Work out the finished part from the listing and answer in its coordinate system (mm). Face numbers are marked on the shaded views. A direction names the side the tool comes from. Coordinates: 2 decimals unless noted, no trailing zeros. Loops run counter-clockwise (first coordinate to the right, second up) from the corner with the lowest first, then second, coordinate; pieces in that order, holes last. Notation, with made-up numbers: M 64,63 L 114,63 A34 cw 114,98 Z; hole C -33.75,10.5 d3. An arc over 180 degrees is marked long. Write each question's results on one line, items separated by ' | '.
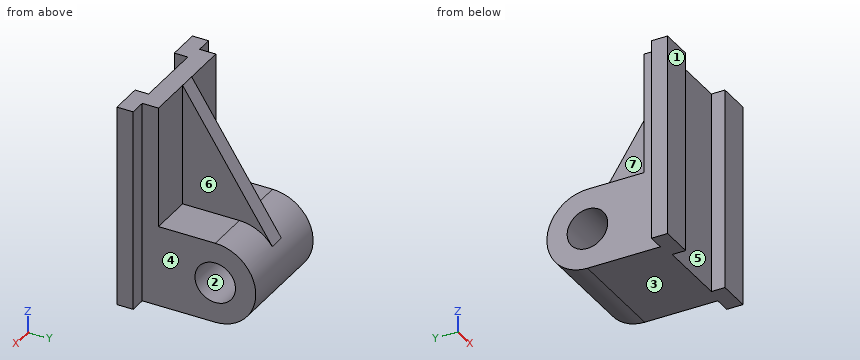
```python
from build123d import *

# Parameters (mm, degrees)
BOSS_EXTRUDE1_DEPTH = 150
SKETCH4_R           = 15
BOSS_EXTRUDE2_DEPTH = 38
RIB1_REACH          = 181.042
SKETCH5_WALL_W      = 482.19756146
SKETCH5_WALL_H      = 12


with BuildPart() as part:
    # Sketch1 → Boss-Extrude1 (new body)
    with BuildSketch(Plane.XY):
        Polygon((-50, 0), (-38, 0), (-38, 12), (38, 12), (38, 0), (50, 0), (50, -12), (26, -12), (26, -2), (-26, -2), (-26, -12), (-50, -12), align=None)
    extrude(amount=BOSS_EXTRUDE1_DEPTH)

    # Sketch4 → Boss-Extrude2 (add, symmetric)
    with BuildSketch(Plane(origin=(0, 0, 0), x_dir=(0, 0, -1), z_dir=(1, 0, 0))):
        with BuildLine():
            Line((0, 12), (0, 54))
            ThreePointArc((0, 54), (-30, 84), (-60, 54))
            Line((-60, 54), (-60, 12))
            Line((-60, 12), (0, 12))
        make_face()
        with Locations((-30, 54)):
            Circle(SKETCH4_R, mode=Mode.SUBTRACT)
    extrude(amount=BOSS_EXTRUDE2_DEPTH, both=True)

    # Sketch5 wall → Rib1 (add, up to next)
    with BuildSketch(Plane(origin=(0, 45.18462462, 98.748424022), x_dir=(0, 0.54350338987, -0.839406972332), z_dir=(0, 0.839406972332, 0.54350338987)), mode=Mode.PRIVATE) as rib1_sk1:
        Rectangle(SKETCH5_WALL_W, SKETCH5_WALL_H)
    rib1_tool1 = extrude(rib1_sk1.sketch, amount=-RIB1_REACH, mode=Mode.PRIVATE) - part.part
    add(rib1_tool1.solids().sort_by_distance((0, 45.18462462, 98.748424022))[0])


solid = part.part
```
1) Find section A-A, the plane x = -35. Give the vertices of the cut face in (y, z).
Check result:
outline: M -12,0 L 54,0 A30 ccw 54,60 L 12,60 L 12,150 L -12,150 Z; hole C 54,30 d30
2) Find section D-D, the plane x = 3. Give the vertices of the cut face in (y, z).
Check result:
outline: M -2,0 L 54,0 A30 ccw 78.37,47.5 L 12,150 L -2,150 Z; hole C 54,30 d30
3) Given pin 1 Ø18 at (y, z) = (54, 30) entering from -X; pin 2 Ø2 at (y, z) = (38.5, 95) entering from +X; pin 3 Ø3 at (x, y) = (-25, 32) entering from +Z; pin 4 Ø4 at (x, z) = (-15, 86.5) entering from -Y, each flat-ended and moving along its own axis, determine where each tip first touches the part or whether it passes through.
Check result:
pin 1: through | pin 2: x = 6 | pin 3: z = 60 | pin 4: y = -2
4) For a pull along Z with two mould halves and no side action, classify the marked faces 1, 2 and 3 as released by +Z, released by -Z, zero draft, split by the parting line, or undercut.
Check result:
face 1: zero draft | face 2: undercut | face 3: released by -Z
5) Straight lines are drawn through the part: probe 1 along Y at (x, z) = (4, 30); probe 2 along X at (y, z) = (-5, 141); probe 3 along X at (y, z) = (33, 115). For each, find the intervals that lie inside material, in ascending order. Write a range as [from, to].
Check result:
probe 1: [-2, 39], [69, 84] | probe 2: [-50, -26], [26, 50] | probe 3: [-6, 6]
6) Find section B-B, the plane z = 30. Give the vertices of the cut face in (x, y).
Check result:
outline: M -50,-12 L -26,-12 L -26,-2 L 26,-2 L 26,-12 L 50,-12 L 50,0 L 38,0 L 38,39 L -38,39 L -38,0 L -50,0 Z; M -38,69 L 38,69 L 38,84 L -38,84 Z
7) Which of the six approach directions +Z, -Z, +X, -X, +Y, -Y give full straight-line access (tool end or side, diameter ignored) to the marked faces 4, 5, 6 and 7?
Check result:
face 4: +Z, -Z, +X, +Y | face 5: +Z, -Z, -Y | face 6: +Z, +X, +Y | face 7: +Z, -X, +Y
8) Find section C-C, the plane y = 43. Give the vertices of the cut face in (x, z).
Check result:
outline: M -38,0 L 38,0 L 38,19.8 L -38,19.8 Z; M -38,40.2 L 38,40.2 L 38,60 L 6,60 L 6,102.12 L -6,102.12 L -6,60 L -38,60 Z
